Check sheet for the modelled part. Datum: model origin and axes. Units: mm. A direction names the side the tool comes from. Round coordinates to 2 decimals unless told otherwise and drop trailing zeros. Order: outer loops, then holes, each group sorted by start corner. A loop starts at its lowest first (then second) coordinate and runs counter-clockwise, first axis right, second up.
Q1. Cross-section at C-C on y = 1.5. Give the number of separate pieces and of enclosed holes in the cut face, then the cut area to 3 significant figures.
Q2. Cross-section at B-B on z = 11.25. Record the cut outline in (x, y), then the cut area to 3 significant figures.
Q3. Mould release check, pull along Y, two halves, no side actions. Record for faces 1 (the flat face through (-19, 4, 27)), 2 (the conical face through (-14.1, 11.84, 26.16)), 3 (the conical face through (-15.421, 12.593, 26.84)): +Y half, -Y half, draft (parallel to the pull), parting line (faces both ways), or undercut.
Q4. Cross-section at A-A on z = 21.75. Record the cut outline in (x, y).
Q5. Scan lines: probe 1 along X at (y, z) = (0, 15); probe 2 along Z at (x, y) = (-4, -8). Record each from-to range of solid material in increasing order.
Q6. Depth check by flat-ended pin: P1, Ø0.8, axis at x = 18.5, z = 25, coming from the -Y side; P2, Ø5, axis at x = -13.5, y = 15, coming from the -Z side; P3, Ø3, axis at x = -9, y = -14.5, coming from the +Z side; P4, Ø8, axis at x = 0, y = 0, coming from the +Z side. Enter the tip coordinate at first touch or a pass-through.
Q7. Set-up check for faces 4 (the flat face through (-5.125, 0, 4)), 5 (the flat face through (18, 6.25, 20)), 6 (the flat face through (11.04, -16.06, 21.95)): record each of +Z, -Z, +X, -X, +Y, -Y from which the full face is reachable in a straight line by a thin tool's end or side.
from build123d import *

# Parameters (mm, degrees)
F0_R      = 20.75
F1_DEPTH  = 6
F3_DEPTH  = 4.75
F4_R      = 3
F5_DEPTH  = 1.25
F6_R      = 20.75
F6_R_2    = 18.25
F7_DEPTH  = 21
F9_W      = 12.5
F9_H      = 5.75
F10_DEPTH = 4.6035718005
F12_DEPTH = 10.25
F13_SIZE  = 1


with BuildPart() as f1:
    # F0 (on Top) → F1 (new body)
    with BuildSketch(Plane.XY):
        Circle(F0_R)
    extrude(amount=F1_DEPTH)

    # F2 (on face) → F3 (cut)
    with BuildSketch(Plane.XY.offset(6)):
        Polygon((5.125, -2.9589201296), (5.125, 2.9589201296), (0, 5.9178402592), (-5.125, 2.9589201296), (-5.125, -2.9589201296), (0, -5.9178402592), align=None)
    extrude(amount=-F3_DEPTH, mode=Mode.SUBTRACT)

    # F4 (on face) → F5 (cut, through all)
    with BuildSketch(Plane.XY.offset(1.25)):
        Circle(F4_R)
    extrude(amount=-F5_DEPTH, mode=Mode.SUBTRACT)

    # F6 (on face) → F7 (join)
    with BuildSketch(Plane.XY.offset(6)):
        Circle(F6_R)
        Circle(F6_R_2, mode=Mode.SUBTRACT)
    extrude(amount=F7_DEPTH)

    # F9 (on offset) → F10 (cut, up to face)
    with BuildSketch(Plane.YZ.offset(20.75)):
        with Locations((0, 19.625)):
            Rectangle(F9_W, F9_H)
    extrude(amount=-F10_DEPTH, mode=Mode.SUBTRACT)

    # F11 (on face) → F12 (cut, through all)
    with BuildSketch(Plane.XY.offset(27)):
        with BuildLine():
            Line((10.3375358146, -15.039875441), (11.7536366111, -17.1001323508))
            ThreePointArc((11.7536366111, -17.1001323508), (16.6770552799, -12.3465917237), (19.7863589374, -6.25))
            Line((19.7863589374, -6.25), (17.1464281995, -6.25))
            ThreePointArc((17.1464281995, -6.25), (14.4276660292, -11.1760884459), (10.3375358146, -15.039875441))
        make_face()
    extrude(amount=-F12_DEPTH, mode=Mode.SUBTRACT)

    # F13
    f13_edges = [f1.edges().sort_by_distance(p)[0] for p in [
        (-18.363693, 9.661122, 27),
        (-16.1512, 8.497131, 27),
        (-20.75, 0, 0),
    ]]
    chamfer(f13_edges, length=F13_SIZE)


solid = f1.part
Results found:
1. separate pieces: 3
1. enclosed holes: 0
1. area: 281 mm2
2. outline: circle Ø41.5 at (0, 0); hole circle Ø36.5 at (0, 0)
2. area: 306 mm2
3. face 1: draft
3. face 2: undercut
3. face 3: parting line
4. outline: (10.34, -15.04) arc R18.25 cw (long way) to (17.15, 6.25) - (19.79, 6.25) arc R20.75 ccw (long way) to (11.75, -17.1) - close
5. probe 1: x = -20.75 to -18.25, 18.25 to 20.75
5. probe 2: z = 0 to 6
6. P1: stops at y = -6.25
6. P2: stops at z = 0
6. P3: stops at z = 26.32
6. P4: stops at z = 1.25
7. face 4: +Z
7. face 5: +X, -Y
7. face 6: +Z, +X
